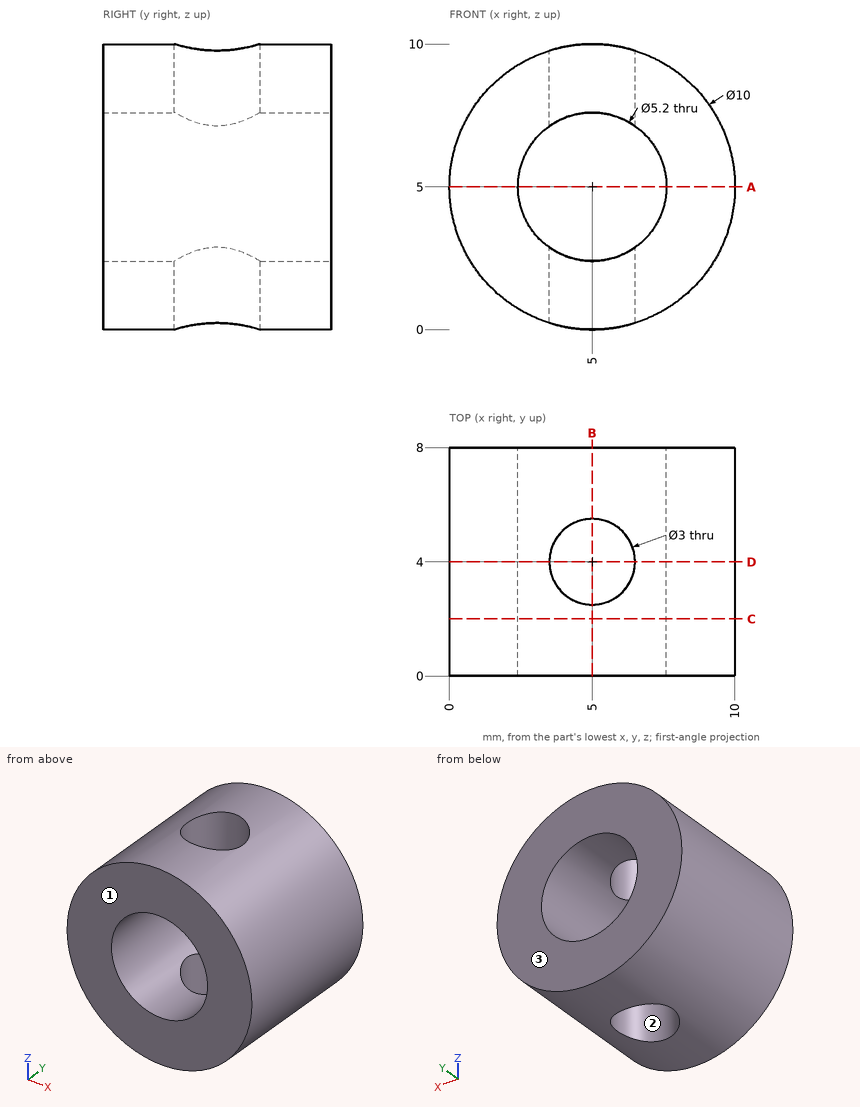
Can you work these out from the drawing? Everything is in mm from the part's minimum corner. Round coordinates to 2 decimals unless told otherwise and drop trailing zeros. Loops run counter-clockwise (first coordinate to the right, second up) from the corner with the lowest first, then second, coordinate; pieces in that order, holes last. Notation, with made-up numbers: (-30, 15.25) - (6, 15.25) arc R13 ccw to (6, 31.25) - close; hole circle Ø8 at (53.5, 12). An arc over 180 degrees is marked (long way). Answer in a Markdown table with one row per item. Add a question column.
Q1. I want a section at D-D on y = 4. List the corners of the cut face in (x, z) for me, and give its area (3 significant figures).
Q2. I need wall thicknesses on L1, parallel to X at y = 3.75, z = 5; L2, parallel to Z at x = 3.25, y = 7.5; L3, parallel to X at y = 5, z = 6.5. Which ranges of each line are inside material? Lowest first, please.
Q3. For pin 1 Ø2 at (x, y) = (5.5, 3.5) entering from -Z; pin 2 Ø1.5 at (y, z) = (2.5, 7) entering from +X, each with a flat end and sliding along its axis, tell me the tip position at first contact or that it passes through.
Q4. I want a section at A-A on z = 5. List the corners of the cut face in (x, y) for me.
Q5. I want a section at C-C on y = 2. List the corners of the cut face in (x, z) for me, and give its area (3 significant figures).
Q6. We'd pull the mould along Y, two halves only. Please class the marked faces 1, 2 and 3: pulls with the +Y half, pulls with the -Y half, needs draft (parallel to the pull), parting line crosses it, or undercut.
Q7. I want a section at B-B on x = 5. List the corners of the cut face in (y, z) for me, and give its area (3 significant figures).
A:
| question | item | result |
|---|---|---|
| 1 | outline | (3.5, 0.23) - (3.5, 2.88) arc R2.6 cw to (3.5, 7.12) - (3.5, 9.77) arc R5 ccw to start; (6.5, 0.23) arc R5 ccw to (6.5, 9.77) - (6.5, 7.12) arc R2.6 cw to (6.5, 2.88) - close |
| 1 | area | 42.4 mm^2 |
| 2 | L1 | 0 to 2.4, 7.6 to 10 |
| 2 | L2 | 0.32 to 3.08, 6.92 to 9.68 |
| 2 | L3 | 0.23 to 2.88, 7.12 to 9.77 |
| 3 | pin 1 | z = 0.01 |
| 3 | pin 2 | x = 9.84 |
| 4 | outline | (0, 0) - (2.4, 0) - (2.4, 8) - (0, 8) - close; (7.6, 0) - (10, 0) - (10, 8) - (7.6, 8) - close |
| 5 | outline | circle Ø10 at (5, 5); hole circle Ø5.2 at (5, 5) |
| 5 | area | 57.3 mm^2 |
| 6 | face 1 | pulls with the -Y half |
| 6 | face 2 | undercut |
| 6 | face 3 | pulls with the +Y half |
| 7 | outline | (0, 0) - (2.5, 0) - (2.5, 2.4) - (0, 2.4) - close; (0, 7.6) - (2.5, 7.6) - (2.5, 10) - (0, 10) - close; (5.5, 0) - (8, 0) - (8, 2.4) - (5.5, 2.4) - close; (5.5, 7.6) - (8, 7.6) - (8, 10) - (5.5, 10) - close |
| 7 | area | 24.0 mm^2 |
